from build123d import *

# Parameters (mm, degrees)
DODANIE_WYCI_GNI_CIE1_DEPTH = 30.2
SZKIC2_R                    = 7.5
WYTNIJ_WYCI_GNI_CIE1_DEPTH  = 94.745879909
ZAOKR_GLENIE1_R             = 2
WYTNIJ_WYCI_GNI_CIE2_REACH  = 87.137


with BuildPart() as part:
    # Szkic1 → Dodanie-wyciągnięcie1 (new body)
    with BuildSketch(Plane(origin=(0, 0, 0), x_dir=(0, 0, -1), z_dir=(1, 0, 0))):
        with BuildLine():
            Line((31.8, 14), (63.5, 14))
            Line((63.5, 14), (63.5, 0))
            Line((63.5, 0), (-63.5, 0))
            Line((-63.5, 0), (-63.5, 14))
            Line((-63.5, 14), (-31.8, 14))
            Line((-31.8, 14), (-31.8, 30.2))
            ThreePointArc((-31.8, 30.2), (0, 62), (31.8, 30.2))
            Line((31.8, 30.2), (31.8, 14))
        make_face()
    extrude(amount=DODANIE_WYCI_GNI_CIE1_DEPTH)

    # Szkic2 → Wytnij-wyciągnięcie1 (cut, through all)
    with BuildSketch(Plane(origin=(30.2, 0, 0), x_dir=(0, 0, -1), z_dir=(1, 0, 0))):
        with Locations((0, 30.2)):
            Circle(SZKIC2_R)
    extrude(amount=-WYTNIJ_WYCI_GNI_CIE1_DEPTH, mode=Mode.SUBTRACT)

    # Zaokrąglenie1
    zaokr_glenie1_edges = [part.edges().sort_by_distance(p)[0] for p in [
        (0, 14, -47.65),
        (15.1, 14, 63.5),
        (15.1, 14, 31.8),
        (15.1, 14, -31.8),
        (15.1, 14, -63.5),
        (30.2, 14, -47.65),
        (30.2, 22.1, -31.8),
        (30.2, 62, 0),
        (30.2, 22.1, 31.8),
        (30.2, 14, 47.65),
        (0, 14, 47.65),
        (0, 22.1, 31.8),
        (0, 62, 0),
        (0, 22.1, -31.8),
    ]]
    fillet(zaokr_glenie1_edges, radius=ZAOKR_GLENIE1_R)

    # Szkic3 → Wytnij-wyciągnięcie2 (cut, up to next)
    with BuildSketch(Plane(origin=(0, 14, 0), x_dir=(1, 0, 0), z_dir=(0, 1, 0)), mode=Mode.PRIVATE) as wytnij_wyci_gni_cie2_sk1:
        with BuildLine():
            Line((8.1, -52.5), (8.1, -42.5))
            ThreePointArc((8.1, -42.5), (15.1, -35.5), (22.1, -42.5))
            Line((22.1, -42.5), (22.1, -52.5))
            ThreePointArc((22.1, -52.5), (15.1, -59.5), (8.1, -52.5))
        make_face()
    wytnij_wyci_gni_cie2_tool1 = extrude(wytnij_wyci_gni_cie2_sk1.sketch, amount=-WYTNIJ_WYCI_GNI_CIE2_REACH, mode=Mode.PRIVATE) & part.part
    # Szkic3 → Wytnij-wyciągnięcie2 (cut, up to next)
    with BuildSketch(Plane(origin=(0, 14, 0), x_dir=(1, 0, 0), z_dir=(0, 1, 0)), mode=Mode.PRIVATE) as wytnij_wyci_gni_cie2_sk2:
        with BuildLine():
            Line((8.1, 42.5), (8.1, 52.5))
            ThreePointArc((8.1, 52.5), (15.1, 59.5), (22.1, 52.5))
            Line((22.1, 52.5), (22.1, 42.5))
            ThreePointArc((22.1, 42.5), (15.1, 35.5), (8.1, 42.5))
        make_face()
    wytnij_wyci_gni_cie2_tool2 = extrude(wytnij_wyci_gni_cie2_sk2.sketch, amount=-WYTNIJ_WYCI_GNI_CIE2_REACH, mode=Mode.PRIVATE) & part.part
    add(wytnij_wyci_gni_cie2_tool1.solids().sort_by_distance((15.1, 14, 47.5))[0], mode=Mode.SUBTRACT)
    add(wytnij_wyci_gni_cie2_tool2.solids().sort_by_distance((15.1, 14, -47.5))[0], mode=Mode.SUBTRACT)


solid = part.part
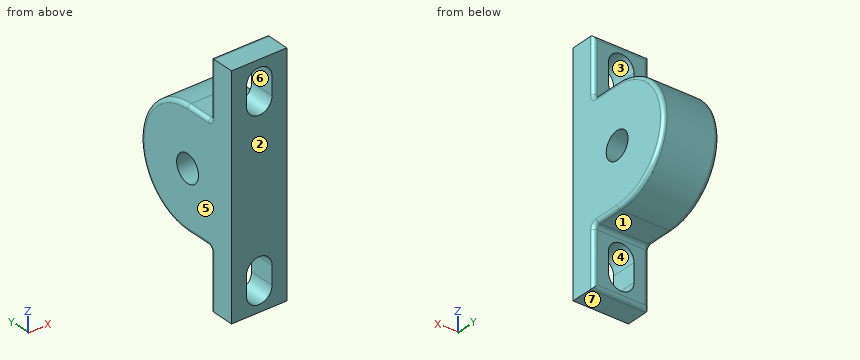
For this review, take the finished solid that the model builds, in its own axes (mm). Face numbers are marked on the shaded views. A direction names the side the tool comes from. Give positions to 0.01 mm unless a question says otherwise; leave off trailing zeros. Loops run counter-clockwise (first coordinate to the right, second up) from the corner with the lowest first, then second, coordinate; pieces in that order, holes last. Notation, with made-up numbers: M -15.5,58 L 38.5,58 A20 cw 38.5,79 Z; hole C 34.5,79 d4. An arc over 180 degrees is marked long. Answer as a JSON object with one key per item and string values. Group by question number.
Q1. For probe 1 along Y at (x, z) = (12, 0); probe 2 along X at (y, z) = (12.5, 44); probe 3 along Z at (x, y) = (5, 26), list the stretches that pass through material, from the lowest coordinate up. Write a range as [from, to].
Q2. Insertion check: P1, Ø4, axis at x = 12, z = -7.5, coming from the +Y side; P2, Ø1.5, axis at x = 22.5, y = 33, coming from the +Z side; P3, Ø12, axis at x = 8, z = -32, coming from the +Y side. Each pin has a flat end and moves straight along its axis. Give the tip position at first contact, or say it passes through.
Q3. Add section C-C on y = 19.5. Give the boundary of the cut face in (x, z), and give its area (3 significant figures).
Q4. Add section A-A on x = 11. Give the boundary of the cut face in (y, z).
Q5. Tool access review of the marked faces 1, 2 and 3: name each direction out of +Z, -Z, +X, -X, +Y, -Y from which nothing blocks a thin tool from reaching the whole face with its end or side.
Q6. Mouldability with a two-part tool opening along X and no side actions: class the marked faces 4, 5, 6 and 7 as +X half, -X half, draft (parallel to the pull), parting line (faces both ways), or undercut.
Q7. Add section D-D on z = 0. Give the boundary of the cut face in (x, y), and give its area (3 significant figures).
Q8. Add section B-B on z = -38. Give the boundary of the cut face in (x, y).
Checked values:
{
 "1": {"probe 1": "[0, 22.7], [37.7, 62]", "probe 2": "[0.06, 8.1], [22.1, 30.14]", "probe 3": "[-31.8, -6.21], [6.21, 31.8]"},
 "2": {"P1": "y = 61.52", "P2": "z = 31.73", "P3": "y = 48.51"},
 "3": {"outline": "M 0,-29.8 A2 ccw 2,-31.8 L 28.2,-31.8 A2 ccw 30.2,-29.8 L 30.2,29.8 A2 ccw 28.2,31.8 L 2,31.8 A2 ccw 0,29.8 Z", "area": "1,920 mm²"},
 "4": {"outline": "M 0,-63.5 L 12,-63.5 A2 ccw 14,-61.5 L 14,-58.17 L 0,-58.17 Z; M 0,-36.83 L 14,-36.83 L 14,-33.8 A2 cw 16,-31.8 L 30.2,-31.8 A31.8 ccw 30.2,31.8 L 16,31.8 A2 cw 14,33.8 L 14,36.83 L 0,36.83 Z; M 0,58.17 L 14,58.17 L 14,61.5 A2 ccw 12,63.5 L 0,63.5 Z; hole C 30.2,0 d15"},
 "5": {"face 1": "-Z, +X, -X, +Y", "face 2": "+Z, -Z, +X, -X, -Y", "face 3": "+Y, -Y"},
 "6": {"face 4": "undercut", "face 5": "-X half", "face 6": "undercut", "face 7": "draft"},
 "7": {"outline": "M 0,0 L 30.2,0 L 30.2,22.7 L 0,22.7 Z; M 0,37.7 L 30.2,37.7 L 30.2,60 A2 ccw 28.2,62 L 2,62 A2 ccw 0,60 Z", "area": "1,420 mm²"},
 "8": {"outline": "M 0,0 L 9.74,0 L 9.74,14 L 2,14 A2 ccw 0,12 Z; M 20.46,0 L 30.2,0 L 30.2,12 A2 ccw 28.2,14 L 20.46,14 Z"}
}
